from build123d import *

# Parameters (mm, degrees)
BOSS_EXTRUDE1_DEPTH = 6.35
SKETCH1_4_W         = 5.585166648
SKETCH1_4_H         = 5.632100821
SKETCH1_4_W_2       = 6.80545516
SKETCH1_4_H_2       = 12.437555982
SKETCH1_4_H_3       = 11.076464949
SKETCH1_4_H_4       = 10.982596602
SKETCH1_4_W_3       = 5.534111201
SKETCH1_4_H_5       = 16.61114729
SKETCH1_4_W_4       = 5.595450485
SKETCH1_4_H_6       = 40.116759918
SKETCH1_4_H_7       = 6.891111662
SKETCH1_4_W_5       = 11.108414189
SKETCH1_4_H_8       = 5.424016142
BOSS_EXTRUDE2_DEPTH = 5.08


with BuildPart() as part:
    # Sketch1 → Boss-Extrude1 (new, symmetric)
    with BuildSketch(Plane.XY):
        Polygon((36.765931583, 20.970924677), (42.300042784, 20.970924677), (42.300042784, -19.145835241), (36.765931583, -19.145835241), (36.765931583, -35.756982531), (29.851375766, -35.756982531), (29.851375766, -48.199580791), (-15.795061386, -48.199580791), (-15.795061386, -35.756982531), (-21.349268481, -35.756982531), (-21.349268481, -24.774385929), (-26.934435129, -24.774385929), (-26.934435129, -13.69792098), (-32.519601777, -13.69792098), (-32.519601777, -1.260364998), (-39.325056937, -1.260364998), (-39.325056937, 4.371735823), (-44.910223585, 4.371735823), (-44.910223585, 15.422486478), (-32.473823981, 15.422486478), (-32.473823981, 9.897989881), (-26.874799511, 9.897989881), (-26.874799511, -6.713303634), (-21.349268481, -6.713303634), (-21.349268481, 68.024806454), (-10.240854292, 68.024806454), (-10.240854292, 15.422486478), (-4.751796061, 15.422486478), (-4.751796061, 38.947796151), (7.735264144, 38.947796151), (7.735264144, 15.422486478), (13.247182022, 15.422486478), (13.247182022, 33.41786203), (24.337202566, 33.41786203), (24.337202566, 9.897989881), (29.851375766, 9.897989881), (29.851375766, 27.862036339), (36.765931583, 27.862036339), align=None)
    extrude(amount=BOSS_EXTRUDE1_DEPTH, both=True)

    # Sketch1_4 → Boss-Extrude2 (add, symmetric)
    with BuildSketch(Plane.XY):
        Polygon((-44.910223585, 15.422486478), (-44.910223585, 4.371735823), (-50.454609627, 4.371735823), (-50.454609627, 20.888501361), (-32.473823981, 20.888501361), (-32.473823981, 15.422486478), align=None)
        with Locations((-42.117640261, 1.555685412)):
            Rectangle(SKETCH1_4_W, SKETCH1_4_H)
        with Locations((-35.922329357, -7.479142989)):
            Rectangle(SKETCH1_4_W_2, SKETCH1_4_H_2)
        with Locations((-29.727018453, -19.236153455)):
            Rectangle(SKETCH1_4_W, SKETCH1_4_H_3)
        with Locations((-24.141851805, -30.26568423)):
            Rectangle(SKETCH1_4_W, SKETCH1_4_H_4)
        Polygon((-15.795061386, -35.756982531), (-15.795061386, -48.199580791), (29.851375766, -48.199580791), (29.851375766, -35.756982531), (36.765931583, -35.756982531), (36.765931583, -53.531928868), (-21.349268481, -53.531928868), (-21.349268481, -35.756982531), align=None)
        with Locations((39.532987184, -27.451408886)):
            Rectangle(SKETCH1_4_W_3, SKETCH1_4_H_5)
        with Locations((45.097768027, 0.912544718)):
            Rectangle(SKETCH1_4_W_4, SKETCH1_4_H_6)
        with Locations((39.532987184, 24.416480508)):
            Rectangle(SKETCH1_4_W_3, SKETCH1_4_H_7)
        Polygon((24.337202566, 9.897989881), (24.337202566, 33.41786203), (36.765931583, 33.41786203), (36.765931583, 27.862036339), (29.851375766, 27.862036339), (29.851375766, 9.897989881), align=None)
        Polygon((7.735264144, 15.422486478), (7.735264144, 38.947796151), (24.337202566, 38.947796151), (24.337202566, 33.41786203), (13.247182022, 33.41786203), (13.247182022, 15.422486478), align=None)
        Polygon((-10.240854292, 15.422486478), (-10.240854292, 68.024806454), (-4.751796061, 68.024806454), (-4.751796061, 44.510136865), (7.735264144, 44.510136865), (7.735264144, 38.947796151), (-4.751796061, 38.947796151), (-4.751796061, 15.422486478), align=None)
        with Locations((-15.795061387, 70.736814525)):
            Rectangle(SKETCH1_4_W_5, SKETCH1_4_H_8)
        Polygon((-32.473823981, 9.897989881), (-32.473823981, 15.422486478), (-26.934435129, 15.422486478), (-26.934435129, 68.024806454), (-21.349268481, 68.024806454), (-21.349268481, -6.713303634), (-26.874799511, -6.713303634), (-26.874799511, 9.897989881), align=None)
    extrude(amount=BOSS_EXTRUDE2_DEPTH, both=True)


solid = part.part
Can you work these out from the model? Positions are in its coordinate system, mm. A direction names the side the tool comes from. Coordinates: 2 decimals unless noted, no trailing zeros. Write each loop counter-clockwise with the first axis right and the second up, starting at its lowest first coordinate (ties: lowest second). Pieces come first, ordered by that corner, then holes. Notation, with made-up numbers: (-32, 29) -> (1, 29) arc R18 cw to (1, 40) -> close; hole circle Ø1 at (49, 21). An arc over 180 degrees is marked (long way). Write item = value, one per line.
(1) Imagine slicing it at A-A (x = -24). Please give me the cut outline in (y, z).
Verdict:
outline = (-35.76, -5.08) -> (-24.77, -5.08) -> (-24.77, -6.35) -> (-6.71, -6.35) -> (-6.71, -5.08) -> (68.02, -5.08) -> (68.02, 5.08) -> (-6.71, 5.08) -> (-6.71, 6.35) -> (-24.77, 6.35) -> (-24.77, 5.08) -> (-35.76, 5.08) -> close
(2) Imagine slicing it at B-B (y = 50). Please give me the cut outline in (x, z), and give its area (3 significant figures).
Verdict:
outline = (-26.93, -5.08) -> (-21.35, -5.08) -> (-21.35, -6.35) -> (-10.24, -6.35) -> (-10.24, -5.08) -> (-4.75, -5.08) -> (-4.75, 5.08) -> (-10.24, 5.08) -> (-10.24, 6.35) -> (-21.35, 6.35) -> (-21.35, 5.08) -> (-26.93, 5.08) -> close
area = 254 mm^2
(3) If I drill on probe 1 along Y at (x, z) = (24, -4.75); probe 2 along Y at (x, z) = (-29.5, 0.75); probe 3 along X at (y, z) = (-30.5, 5.25), over which ranges is the centre line in solid material (lowest first)?
Verdict:
probe_1 = -53.53 to 38.95
probe_2 = -24.77 to 15.42
probe_3 = -21.35 to 36.77
(4) For pin 1 (6 mm diameter, centred on x = 41, y = -24.5, fed in from -Z); pin 2 (0.6 mm diameter, centred on x = -23.5, z = -5.5, fed in from -Y); pin 3 (3 mm diameter, centred on y = 29.5, z = 3.5, fed in from -X), each with a flat end and sliding along its axis, tell me the tip position at first contact or that it passes through.
Verdict:
pin_1 = -5.08
pin_2 = -24.77
pin_3 = -26.93
(5) Imagine slicing it at C-C (y = 1). Please give me the cut outline in (x, z), and give its area (3 significant figures).
Verdict:
outline = (-44.91, -5.08) -> (-39.33, -5.08) -> (-39.33, -6.35) -> (-26.87, -6.35) -> (-26.87, -5.08) -> (-21.35, -5.08) -> (-21.35, -6.35) -> (42.3, -6.35) -> (42.3, -5.08) -> (47.9, -5.08) -> (47.9, 5.08) -> (42.3, 5.08) -> (42.3, 6.35) -> (-21.35, 6.35) -> (-21.35, 5.08) -> (-26.87, 5.08) -> (-26.87, 6.35) -> (-39.33, 6.35) -> (-39.33, 5.08) -> (-44.91, 5.08) -> close
area = 1,140 mm^2
(6) On a 3-axis mill with a long thin cutter (end or side, diameter ignored), from which of +Z, -Z, +X, -X, +Y, -Y can I reach the whole of each face in a straight line? I mean faces 4 (the face through (-42, 20.889, 0)), 5 (the face through (36.766, 31, 0)), 6 (the face through (-42, -1.26, 0)), 7 (the face through (45, 1, -5.08)), 8 (the face through (-30, -19, 5.08)). Say none if no direction works.
Verdict:
face_4 = +Z, -Z, -X, +Y
face_5 = +Z, -Z, +X, +Y
face_6 = +Z, -Z, -X, -Y
face_7 = -Z, +X, +Y, -Y
face_8 = +Z, -X, -Y
(7) Thinking about a two-plate mould opening in X: for faces 1 (the face through (-30, -24.774, 0)), 2 (the face through (-21.349, 71, 0)), 3 (the face through (-5, 42, 5.08)), which applies, +X half, -X half, draft (parallel to the pull), parting line (faces both ways), or undercut?
Verdict:
face_1 = draft
face_2 = -X half
face_3 = undercut
